Check sheet for the modelled part. Datum: model origin and axes. Units: mm. Round coordinates to 2 decimals unless told otherwise and drop trailing zeros. Loops run counter-clockwise (first coordinate to the right, second up) from the corner with the lowest first, then second, coordinate; pieces in that order, holes last. Notation, with made-up numbers: (-30, 73) -> (8, 73) arc R19 cw to (8, 103) -> close; hole circle Ø2 at (70, 66). An arc over 180 degrees is marked (long way). Return JSON: item names as keys, results as strings.
from build123d import *

# Parameters (mm, degrees)
BOSS_EXTRU_1_DEPTH           = 215
ESQUISSE2_W                  = 13
ESQUISSE2_H                  = 3
ENL_V_MAT_EXTRU_1_DEPTH      = 5
ESQUISSE3_W                  = 12
ESQUISSE3_H                  = 6
ENL_V_MAT_EXTRU_2_DEPTH      = 217.309962785
ESQUISSE4_R                  = 1
ENL_V_MAT_EXTRU_3_DEPTH      = 10
ENL_V_MAT_EXTRU_4_DEPTH      = 217.309962785
ENL_V_MAT_EXTRU_4_DEPTH_BACK = 217.309962785
ESQUISSE5_W                  = 11
ESQUISSE5_H                  = 6


with BuildPart() as part:
    # Esquisse1 → Boss.-Extru.1 (new body)
    with BuildSketch(Plane(origin=(0, 0, 0), x_dir=(1, 0, 0), z_dir=(0, 1, 0))):
        Polygon((0, 0), (0, 6), (17.5, 6), (17.5, 3), (23, 3), (23, 0), align=None)
    extrude(amount=BOSS_EXTRU_1_DEPTH)

    # Esquisse2 → Enlèv. mat.-Extru.1 (cut)
    with BuildSketch(Plane(origin=(0, 215, 0), x_dir=(1, 0, 0), z_dir=(0, 1, 0))):
        with Locations((6.5, 1.5)):
            Rectangle(ESQUISSE2_W, ESQUISSE2_H)
    extrude(amount=-ENL_V_MAT_EXTRU_1_DEPTH, mode=Mode.SUBTRACT)

    # Esquisse3 → Enlèv. mat.-Extru.2 (cut, through all)
    with BuildSketch(Plane.XY):
        with Locations((11, 178)):
            Rectangle(ESQUISSE3_W, ESQUISSE3_H)
    extrude(amount=-ENL_V_MAT_EXTRU_2_DEPTH, mode=Mode.SUBTRACT)

    # Esquisse4 → Enlèv. mat.-Extru.3 (cut)
    with BuildSketch(Plane(origin=(0, 215, 0), x_dir=(1, 0, 0), z_dir=(0, 1, 0))):
        with Locations(Location((14.5, 3, 0), (0, 0, 270))):
            Circle(ESQUISSE4_R)
    extrude(amount=-ENL_V_MAT_EXTRU_3_DEPTH, mode=Mode.SUBTRACT)

    # Esquisse5 → Enlèv. mat.-Extru.4 (cut, two sides: drawn at the far end of the back side and taken through both)
    with BuildSketch(Plane(origin=(0, 0, -6), x_dir=(-1, 0, 0), z_dir=(0, 0, -1)).offset(-ENL_V_MAT_EXTRU_4_DEPTH_BACK)):
        with Locations((-11.5, 52)):
            Rectangle(ESQUISSE5_W, ESQUISSE5_H)
    extrude(amount=ENL_V_MAT_EXTRU_4_DEPTH + ENL_V_MAT_EXTRU_4_DEPTH_BACK, mode=Mode.SUBTRACT)


solid = part.part
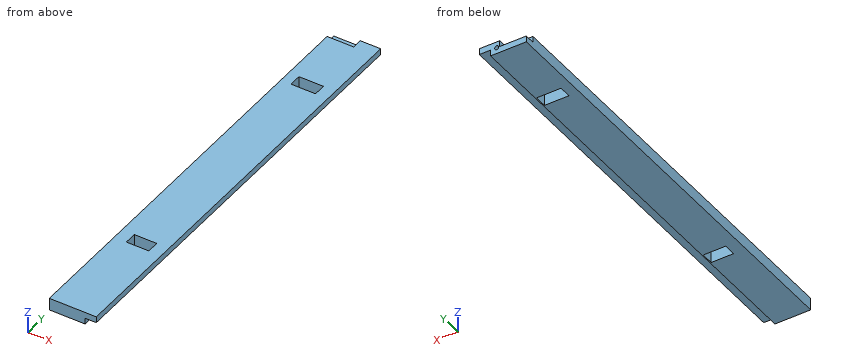
Q1. Section check B-B (y = 134.5). Record the boundary of the cut face in (x, z), then the cut area to 4 significant figures.
Results list:
{"outline": "(0, -6) -> (17.5, -6) -> (17.5, -3) -> (23, -3) -> (23, 0) -> (0, 0) -> close", "area": "121.5 mm^2"}
Q2. Material ranges on line 1 (Y direction, x = 8.75, z = -1.15); line 2 (Y direction, x = 9.75, z = -5.2); line 3 (Y direction, x = 5.75, z = -1.85), recorded low to high.
Results list:
{"line 1": "0 to 49, 55 to 175, 181 to 210", "line 2": "0 to 49, 55 to 175, 181 to 215", "line 3": "0 to 175, 181 to 210"}
Q3. Section check A-A (x = 9.5). Record the boundary of the cut face in (y, z).
Results list:
{"outline": "(0, -6) -> (49, -6) -> (49, 0) -> (0, 0) -> close; (55, -6) -> (175, -6) -> (175, 0) -> (55, 0) -> close; (181, -6) -> (215, -6) -> (215, -3) -> (210, -3) -> (210, 0) -> (181, 0) -> close"}
Q4. Go/stop test with flat-tipped pins: pin 1 (4 mm diameter, centred on x = 6, y = 213, fed in from +Z); pin 2 (0.9 mm diameter, centred on y = 109, z = -4, fed in from +X); pin 3 (1.5 mm diameter, centred on x = 18.5, y = 65, fed in from -Z). Record where each tip stops, or that it passes through.
Results list:
{"pin 1": "z = -3", "pin 2": "x = 17.5", "pin 3": "z = -3"}
Q5. Section check C-C (x = 19.75). Record the boundary of the cut face in (y, z), then the cut area to 3 significant figures.
Results list:
{"outline": "(0, -3) -> (215, -3) -> (215, 0) -> (0, 0) -> close", "area": "645 mm^2"}
